```python
from build123d import *

# Parameters (mm, degrees)
F0_W          = 152.4
F0_H          = 101.6
F1_ANGLE_BACK = 22.5
F1_ANGLE      = 45
F2_T          = -2.54
F3_R          = 5.08
F4_W          = 39.3600463867
F4_H          = 20.9691906348
F5_DEPTH      = 25.4


with BuildPart() as f1:
    # F0 (on Top) → F1 (revolve)
    with BuildSketch(Plane.XY, mode=Mode.PRIVATE) as f1_sk:
        with Locations((-76.2, -50.8)):
            Rectangle(F0_W, F0_H)
    revolve(f1_sk.sketch.rotate(Axis((0, -50.8, 0), (0, 1, 0)), -F1_ANGLE_BACK), axis=Axis((0, -50.8, 0), (0, 1, 0)), revolution_arc=F1_ANGLE)

    # F2
    f2_openings = [f1.faces().sort_by_distance(p)[0] for p in [
        (-70.39962, -50.8, 29.160478),
    ]]
    offset(amount=F2_T, openings=f2_openings)

    # F3
    f3_edges = [f1.edges().sort_by_distance(p)[0] for p in [
        (-71.361692, -99.06, -26.809705),
        (-149.854618, -99.06, 1.270046),
        (-139.404714, -50.8, -54.994047),
        (-71.361692, -2.54, -26.809705),
        (-149.854618, -2.54, 1.270046),
    ]]
    fillet(f3_edges, radius=F3_R)

    # F4 (on face) → F5 (cut)
    with BuildSketch(Plane.XZ.offset(101.6)):
        with Locations((-98.6861884594, 1.2850291096)):
            Rectangle(F4_W, F4_H)
    extrude(amount=-F5_DEPTH, mode=Mode.SUBTRACT)


solid = f1.part
```
Part model, mm, in its own coordinate system. A direction names the side the tool comes from. Round coordinates to 2 decimals unless told otherwise and drop trailing zeros. Order: outer loops, then holes, each group sorted by start corner. A loop starts at its lowest first (then second) coordinate and runs counter-clockwise, first axis right, second up. Notation, with made-up numbers: M 31.25,-15 L 83.25,-15 A29 cw 83.25,21 Z; hole C 26,70 d4. An arc over 180 degrees is marked long. Put each result on its own line as item: value. Start each with the question number.
1. Two-plate mould, pull along Y, no slides. Class faces 3 (the face through (-106, -101.6, 15)), 4 (the face through (-101, -2.54, 7)), 5 (the face through (-75.943, -99.481, 31.457)), 6 (the face through (-69.851, -50.195, -26.184)): +Y half, -Y half, draft (parallel to the pull), parting line (faces both ways), or undercut.
2. Drill centre lines: probe 1 along Y at (x, z) = (-83.5, -13); probe 2 along X at (y, z) = (-40.5, -7); probe 3 along X at (y, z) = (-83, -51). Where is each one in solid material? Low to high. Write a range as [from, to].
3. Drop flat-ended pins along their axis: pin 1 (6 mm diameter, centred on y = -52, z = 4.5, fed in from -X); pin 2 (5 mm diameter, centred on y = -32, z = -19, fed in from +X); pin 3 (2 mm diameter, centred on x = -93.5, y = -100, fed in from -Z). Give the stop position or say it passes through.
4. Tool access for faces 1 (the face through (-105, -99.06, 17)), 2 (the face through (-71.39, -50.09, -29.57)): list every direction of +Z, -Z, +X, -X, +Y, -Y with a clear straight run to the whole face (end or side of a thin tool).
5. Slice it at A-A on y = -61. List the corners of the cut face in (x, z), then the cut area to 3 significant figures.
Findings:
1. face 3: -Y half
1. face 4: undercut
1. face 5: draft
1. face 6: undercut
2. probe 1: [-101.6, -99.06], [-2.54, 0]
2. probe 2: [-152.24, -149.7], [-23.54, -16.9]
2. probe 3: [-143.61, -140.79], [-129.76, -123.12]
3. pin 1: x = -152.39
3. pin 2: x = -39.83
3. pin 3: z = -39.14
4. face 1: none
4. face 2: -Z, +X, +Y, -Y
5. outline: M -141.28,-49.98 A149.86 cw -138.45,57.35 L -140.8,58.32 A152.4 ccw -140.8,-58.32 L 0,0 L -3.32,1.37 L -134.55,-52.98 A5.08 cw Z
5. area: 685 mm2
